Part model, mm, in its own coordinate system. A direction names the side the tool comes from. Give positions to 0.01 mm unless a question says otherwise; leave off trailing zeros. Write each loop counter-clockwise with the first axis right and the second up, starting at its lowest first coordinate (ties: lowest second). Pieces come first, ordered by that corner, then holes.
from build123d import *

# Parameters (mm, degrees)
SKETCH_1_W                  = 47
SKETCH_1_H                  = 21
EXTRUDE_1_DEPTH             = 70
SHELL_1_T                   = -1
SKETCH_2_W                  = 29
SKETCH_2_H                  = 1
EXTRUDE_2_DEPTH             = 26
SKETCH_3_W                  = 45
SKETCH_3_H                  = 1
EXTRUDE_3_DEPTH             = 7
HOLE_WIZARD_10_0_10_1_D     = 10
HOLE_WIZARD_10_0_10_1_DEPTH = 1
HOLE_WIZARD_3_5_3_5_1_D     = 3.5
HOLE_WIZARD_M3_1_D          = 2.5
CHAMFER_1_SIZE              = 5
FILLET_1_R                  = 0.5


with BuildPart() as part:
    # 草图1 → 凸台-拉伸1 (new body)
    with BuildSketch(Plane(origin=(0, 0, 0), x_dir=(1, 0, 0), z_dir=(0, 1, 0))):
        with Locations((-23.5, 10.5)):
            Rectangle(SKETCH_1_W, SKETCH_1_H)
    extrude(amount=EXTRUDE_1_DEPTH)

    # 抽壳1
    shell_1_openings = [part.faces().sort_by_distance(p)[0] for p in [
        (-23.5, 70, -10.5),
        (-23.5, 35, 0),
        (-23.5, 35, -21),
    ]]
    offset(amount=SHELL_1_T, openings=shell_1_openings, kind=Kind.INTERSECTION)

    # 草图2 → 凸台-拉伸2 (add)
    with BuildSketch(Plane.XY):
        with Locations((-31.5, 0.5)):
            Rectangle(SKETCH_2_W, SKETCH_2_H)
    extrude(amount=EXTRUDE_2_DEPTH)

    # 草图3 → 凸台-拉伸3 (add)
    with BuildSketch(Plane(origin=(0, 0, -21), x_dir=(-1, 0, 0), z_dir=(0, 0, -1))):
        with Locations((23.5, 0.5)):
            Rectangle(SKETCH_3_W, SKETCH_3_H)
    extrude(amount=EXTRUDE_3_DEPTH)

    # Ø10.0 (10) 直径槽口1
    with Locations(Plane(origin=(0, 0, 0), x_dir=(0, 0, -1), z_dir=(1, 0, 0))):
        with Locations((10.5, 60)):
            Hole(HOLE_WIZARD_10_0_10_1_D / 2, depth=HOLE_WIZARD_10_0_10_1_DEPTH)

    # Ø3.5 (3.5) 直径槽口1 (through all)
    with Locations(Plane.ZY.offset(47)):
        with Locations((-10.5, 60)):
            Hole(HOLE_WIZARD_3_5_3_5_1_D / 2)

    # M3 螺纹孔1 (through all)
    with Locations(Plane(origin=(0, 1, 0), x_dir=(1, 0, 0), z_dir=(0, 1, 0))):
        with Locations((-39, -23), (-24, -23), (-24, 25), (-39, 25)):
            Hole(HOLE_WIZARD_M3_1_D / 2)

    # 倒角1
    chamfer_1_edges = [part.edges().sort_by_distance(p)[0] for p in [
        (-46.5, 70, 0),
        (-46.5, 70, -21),
        (-0.5, 70, 0),
        (-46, 0.5, 26),
        (-17, 0.5, 26),
        (-1, 0.5, -28),
        (-46, 0.5, -28),
        (-0.5, 70, -21),
    ]]
    chamfer(chamfer_1_edges, length=CHAMFER_1_SIZE)

    # 圆角1
    fillet_1_edges = [part.edges().sort_by_distance(p)[0] for p in [
        (-17, 0.5, 0),
        (-47, 0, -10.5),
        (0, 0, -10.5),
    ]]
    fillet(fillet_1_edges, radius=FILLET_1_R)


solid = part.part
1) Flat gauge pins, fed straight in: P1, Ø6, axis at y = 60, z = -10.5, coming from the +X side; P2, Ø0.5, axis at y = 0.5, z = 12.5, coming from the +X side; P3, Ø0.8, axis at x = -46.5, y = 17, coming from the +Z side. Where does each tip first touch, or does it go through?
Check result:
P1: stops at x = -46
P2: stops at x = -17
P3: stops at z = 0
2) Mould opens along X. For faces 1 (the flat face through (-23, 1, -7)), 2 (the flat face through (-3.5, 0.5, -25.5)), 3 (the flat face through (-43.5, 0.5, 23.5)) say: +X half, -X half, draft (parallel to the pull), parting line (faces both ways), or undercut.
Check result:
face 1: undercut
face 2: +X half
face 3: -X half
3) Saw through at D-D (z = -10.5). Write the cut outline in (x, y).
Check result:
outline: (-47, 0.5) arc R0.5 ccw to (-46.5, 0) - (-0.5, 0) arc R0.5 ccw to (0, 0.5) - (0, 55) - (-1, 55) - (-1, 1) - (-46, 1) - (-46, 58.25) - (-47, 58.25) - close; (-47, 61.75) - (-46, 61.75) - (-46, 70) - (-47, 70) - close; (-1, 65) - (0, 65) - (0, 70) - (-1, 70) - close
4) Drill centre lines: L1, parallel to Z at x = -39, y = 0.5; L2, parallel to X at y = 21.5, z = -15.5; L3, parallel to X at y = 0.8, z = -25. Where is each one in solid material? Low to high.
Check result:
L1: z = -28 to -26.25, -23.75 to 21.75, 24.25 to 26
L2: x = -47 to -46, -1 to 0
L3: x = -44 to -40.25, -37.75 to -25.25, -22.75 to -3
5) Saw through at C-C (x = -39). Write the cut outline in (y, z), and give its area (3 significant figures).
Check result:
outline: (0, -28) - (1, -28) - (1, -26.25) - (0, -26.25) - close; (0, -23.75) - (1, -23.75) - (1, 21.75) - (0, 21.75) - close; (0, 24.25) - (1, 24.25) - (1, 26) - (0, 26) - close
area: 49.0 mm2
6) Saw through at B-B (z = 23). Write the cut outline in (x, y).
Check result:
outline: (-44, 0) - (-40.25, 0) - (-40.25, 1) - (-44, 1) - close; (-37.75, 0) - (-25.25, 0) - (-25.25, 1) - (-37.75, 1) - close; (-22.75, 0) - (-19, 0) - (-19, 1) - (-22.75, 1) - close
7) 3-axis set-ups, long thin cutter, end or side, ignore diameter. For faces 4 (the flat face through (-43.5, 0.5, -25.5)), 5 (the flat face through (-1, 35, -10)), 6 (the cylindrical face through (-0.507, 64.216, -7.812)): which of +Z, -Z, +X, -X, +Y, -Y reach the whole face in a straight line?
Check result:
face 4: -Z, -X, +Y, -Y
face 5: +Z, -Z, +Y
face 6: +X
8) Saw through at A-A (y = 40). Write the cut outline in (x, z), and give its area (3 significant figures).
Check result:
outline: (-47, -21) - (-46, -21) - (-46, 0) - (-47, 0) - close; (-1, -21) - (0, -21) - (0, 0) - (-1, 0) - close
area: 42.0 mm2
